Check sheet for the modelled part. Datum: model origin and axes. Units: mm. A direction names the side the tool comes from. Give positions to 0.01 mm unless a question says otherwise; leave off trailing zeros. Loops run counter-clockwise (first coordinate to the right, second up) from the corner with the lowest first, then second, coordinate; pieces in that order, holes last.
```python
from build123d import *

# Parameters (mm, degrees)
SKETCH1_W           = 21
SKETCH1_H           = 26
SKETCH1_W_2         = 28
SKETCH1_H_2         = 6
BOSS_EXTRUDE1_START = 26
SKETCH2_W           = 13.5
SKETCH2_H           = 13.5
BOSS_EXTRUDE1_DEPTH = 36.5


with BuildPart() as part:
    # Sketch1 → Revolve1 (revolve)
    with BuildSketch(Plane.XY, mode=Mode.PRIVATE) as revolve1_sk:
        with Locations((217.1, 39)):
            Rectangle(SKETCH1_W, SKETCH1_H)
        Polygon((82.6, 52.5), (82.6, 26), (206.6, 26), (206.6, 52), (206.6, 53), (82.6, 53), align=None)
        Polygon((80.1, 52), (80.1, 26), (82.6, 26), (82.6, 52.5), (80.1, 52.5), align=None)
        Polygon((0, 42), (0, 26), (80.1, 26), (80.1, 52), (0, 52), align=None)
        Polygon((-2, 32), (-2, 26), (0, 26), (0, 42), (-2, 42), align=None)
        with Locations((-16, 29)):
            Rectangle(SKETCH1_W_2, SKETCH1_H_2)
    revolve(revolve1_sk.sketch.rotate(Axis((-30, 26, 0), (1, 0, 0)), 180), axis=Axis((-30, 26, 0), (1, 0, 0)))

    # Sketch2 → Boss-Extrude1 (add, symmetric)
    with BuildSketch(Plane(origin=(0, 0, 0), x_dir=(1, 0, 0), z_dir=(0, 1, 0)).offset(BOSS_EXTRUDE1_START)):
        with Locations((214.1, 0)):
            Rectangle(SKETCH2_W, SKETCH2_H)
    extrude(amount=BOSS_EXTRUDE1_DEPTH, both=True)


solid = part.part
```
(1) Access from +Z, -Z, +X, -X, +Y, -Y to the whole of each face (thin tool, end or side, straight path). Record for faces 1 (the face through (80.1, 6.5, 17.5)), 2 (the face through (227.6, 26, 0)), 3 (the face through (206.6, 11.9, -22.1)).
(2) Section check B-B on y = 26. Record the boundary of the cut face in (x, z).
(3) Material ranges on line 1 (X direction, y = 25, z = 18); line 2 (X direction, y = 16, z = 5); line 3 (Y direction, x = 65, z = 22), recorded low to high.
(4) Gauge pin test, flat ends, axial feed: pin 1 Ø12.5 at (x, y) = (217, 57.5) entering from -Z; pin 2 Ø6 at (y, z) = (31.5, -9) entering from -X; pin 3 Ø6 at (y, z) = (12, 20) entering from -X. Record the tip position at first contact, or that the pin passes through.
(5) Section check D-D on y = -5. Record the boundary of the cut face in (x, z), plus the area to 3 significant figures.
(6) Section check A-A on x = 212.5. Record the boundary of the cut face in (y, z).
Computed values:
1. face 1: -X
1. face 2: +Z, -Z, +X, +Y, -Y
1. face 3: none
2. outline: (-30, -6) - (-2, -6) - (-2, -16) - (0, -16) - (0, -26) - (80.1, -26) - (80.1, -26.5) - (82.6, -26.5) - (82.6, -27) - (206.6, -27) - (206.6, -26) - (227.6, -26) - (227.6, 26) - (206.6, 26) - (206.6, 27) - (82.6, 27) - (82.6, 26.5) - (80.1, 26.5) - (80.1, 26) - (0, 26) - (0, 16) - (-2, 16) - (-2, 6) - (-30, 6) - close
3. line 1: x = 0 to 227.6
3. line 2: x = -2 to 227.6
3. line 3: y = 12.14 to 39.86
4. pin 1: stops at z = -6.75
4. pin 2: stops at x = -2
4. pin 3: stops at x = 0
5. outline: (207.35, -6.75) - (220.85, -6.75) - (220.85, 6.75) - (207.35, 6.75) - close
5. area: 182 mm2
6. outline: (-10.5, -6.75) - (0.89, -6.75) arc R26 ccw to (51.11, -6.75) - (62.5, -6.75) - (62.5, 6.75) - (51.11, 6.75) arc R26 ccw to (0.89, 6.75) - (-10.5, 6.75) - close
